from build123d import *

# Parameters (mm, degrees)
SKETCH1_R           = 1.9
BOSS_EXTRUDE1_DEPTH = 4
BOSS_EXTRUDE2_DEPTH = 4
FILLET1_R           = 3
FILLET2_R           = 1


with BuildPart() as part:
    # Sketch1 → Boss-Extrude1 (new body)
    with BuildSketch(Plane.XY):
        with BuildLine():
            Line((16.350014, -56.012494518), (14.404736199, -49.348288471))
            ThreePointArc((14.404736199, -49.348288471), (15.780421817, -45.505146042), (19.860711038, -45.621311922))
            ThreePointArc((19.860711038, -45.621311922), (23.789076326, -47.057783014), (27.830450892, -45.979453446))
            ThreePointArc((27.830450892, -45.979453446), (0, 49.65), (-27.830450892, -45.979453446))
            ThreePointArc((-27.830450892, -45.979453446), (-23.789076326, -47.057783014), (-19.860711038, -45.621311922))
            ThreePointArc((-19.860711038, -45.621311922), (-15.780421817, -45.505146042), (-14.404736199, -49.348288471))
            Line((-14.404736199, -49.348288471), (-16.350014, -56.012494518))
            ThreePointArc((-16.350014, -56.012494518), (0, 58.35), (16.350014, -56.012494518))
        make_face()
        with Locations((17.740527432, -48.374572984)):
            Circle(SKETCH1_R, mode=Mode.SUBTRACT)
        with Locations((-17.740527432, -48.374572984)):
            Circle(SKETCH1_R, mode=Mode.SUBTRACT)
    extrude(amount=BOSS_EXTRUDE1_DEPTH)

    # Sketch2 → Boss-Extrude2 (add)
    with BuildSketch(Plane(origin=(0, 0, 0), x_dir=(-1, 0, 0), z_dir=(0, 0, -1))):
        with BuildLine():
            Line((23, 40.733405839), (24.5, 43.498463103))
            ThreePointArc((24.5, 43.498463103), (0, 49.65), (-24.5, 43.498463103))
            Line((-24.5, 43.498463103), (-23, 40.733405839))
            ThreePointArc((-23, 40.733405839), (0, 46.778310692), (23, 40.733405839))
        make_face()
    extrude(amount=-BOSS_EXTRUDE2_DEPTH)

    # Fillet1
    fillet1_edges = [part.edges().sort_by_distance(p)[0] for p in [
        (-24.5, 43.498463103, 2),
        (24.5, 43.498463103, 2),
    ]]
    fillet(fillet1_edges, radius=FILLET1_R)

    # Fillet2
    fillet2_edges = [part.edges().sort_by_distance(p)[0] for p in [
        (-23, 40.733405839, 2),
        (23, 40.733405839, 2),
    ]]
    fillet(fillet2_edges, radius=FILLET2_R)


solid = part.part
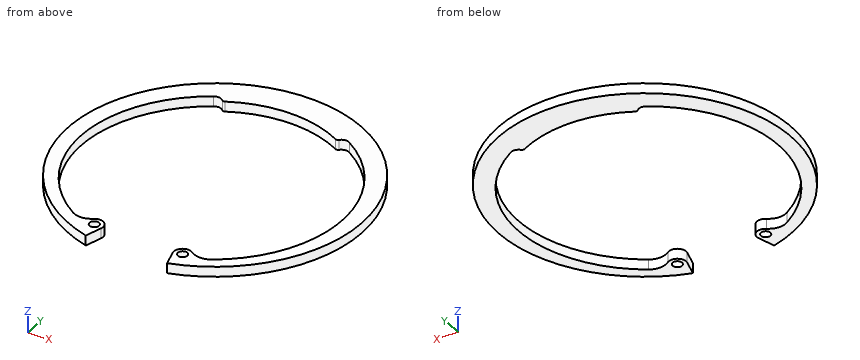
The listing builds one solid part. Answer for the finished solid, in the listing's coordinates (mm). Round coordinates to 2 decimals unless told otherwise and drop trailing zeros. Write each loop counter-clockwise with the first axis right and the second up, starting at its lowest first coordinate (ties: lowest second). Pieces come first, ordered by that corner, then holes. Notation, with made-up numbers: (84.25, 84.25) - (142.25, 84.25) arc R18 cw to (142.25, 111.25) - close; hole circle Ø10 at (22.25, 29.25). An arc over 180 degrees is marked (long way). Use one line per item in the form item = value. Start each with the question number.
Item 1: A flat-ended cylindrical pin translates along its axis: pin 1 Ø1 at (x, z) = (7, 3.5) entering from +Y. Find the tip coordinate at first contact, or state that the pin passes through.
Item 2: A cutting plane is placed at A-A (y = -2.5). Write down the section's boundary in (x, z), plus the area to 3 significant figures.
Item 3: A cutting plane is placed at B-B (x = 0). Write down the section's boundary in (y, z), plus the area to 3 significant figures.
Item 4: A cutting plane is placed at C-C (y = -41.5). Write down the section's boundary in (x, z), plus the area to 3 significant figures.
Item 5: Find the intervals of material crossed by line 1 (Y direction, x = -18, z = 3.85); line 2 (Y direction, x = -39, z = 1.7) (3 decimals); line 3 (X direction, y = -37, z = 2.1), in increasing order. Write a range as [from, to].
Item 6: A cutting plane is placed at D-D (z = 0.8). Give the number of separate pieces and of enclosed holes in the cut face, plus the area to 3 significant figures.
The answers:
q1.pin_1 = 57.99
q2.outline = (-58.3, 0) - (-51.86, 0) - (-51.86, 4) - (-58.3, 4) - close; (51.86, 0) - (58.3, 0) - (58.3, 4) - (51.86, 4) - close
q2.area = 51.5 mm^2
q3.outline = (46.78, 0) - (58.35, 0) - (58.35, 4) - (46.78, 4) - close
q3.area = 46.3 mm^2
q4.outline = (-41.02, 0) - (-33.86, 0) - (-33.86, 4) - (-41.02, 4) - close; (33.86, 0) - (41.02, 0) - (41.02, 4) - (33.86, 4) - close
q4.area = 57.3 mm^2
q5.line_1 = [-55.5, -50.26], [-46.49, -44.91], [43.18, 55.5]
q5.line_2 = [-43.402, -36.404], [31.975, 43.402]
q5.line_3 = [-45.12, -38.47], [38.47, 45.12]
q6.separate_pieces = 1
q6.enclosed_holes = 2
q6.area = 2,320 mm^2
